Here's the drawing with two shaded views (mm, measured from the low corner). I have some questions. A direction names the side the tool comes from. Coordinates: 2 decimals unless noted, no trailing zeros. Write each loop counter-clockwise with the first axis right and the second up, starting at its lowest first coordinate (ties: lowest second). Pieces come first, ordered by that corner, then holes. Notation, with made-up numbers: (23, 38.5) -> (79, 38.5) arc R27 ccw to (79, 65.5) -> close; hole circle Ø6 at (11.5, -33). An arc over 180 degrees is marked (long way). Answer in a Markdown table with one row per item. Add a question column.
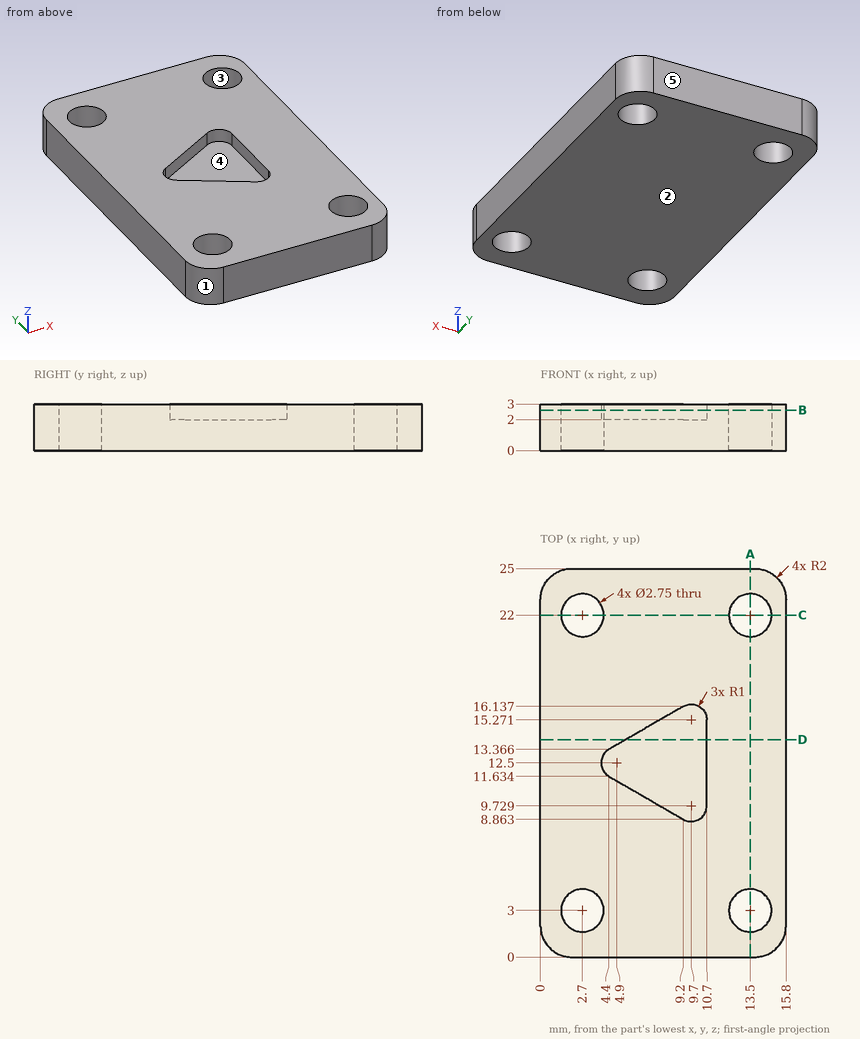
Q1. Imagine slicing it at C-C on y = 22. Please give me the cut outline in (x, z) (1 decimal).
Q2. Imagine slicing it at A-A on x = 13.5. Please give me the cut outline in (y, z) (1 decimal), plus the area to 3 significant figures.
Q3. For the marked faces 4 and 5, which set-ups out of +Z, -Z, +X, -X, +Y, -Y let a thin tool reach every point of the face, with its end or its side?
Q4. I'm going to push a flat-ended pin straight in: P1, Ø1.6, axis at x = 13.5, y = 3, coming from the -Z side. Where does the tip first touch, or does it pass through?
Q5. Imagine slicing it at B-B on z = 2.6. State how many separate pieces and enclosed holes the cut face has, plus the area to 3 significant figures.
Q6. I need wall thicknesses on line 1 (Y direction, x = 2.7, z = 1.8) (1 decimal); line 2 (Y direction, x = 2.25, z = 1.5); line 3 (X direction, y = 23.25, z = 0.4) (1 decimal). Which ranges of each line are inside material? Lowest first, please. Write a range as [from, to].
Q7. Imagine slicing it at D-D on y = 14. Please give me the cut outline in (x, z).
Q8. If we mould it in two halves opening along Y, with no side actions, what happens to the marked faces 1, 2 and 3? For each: pulls with the +Y half, pulls with the -Y half, needs draft (parallel to the pull), parting line crosses it, or undercut.
Result sheet:
| question | item | result |
|---|---|---|
| 1 | outline | (0, 0) -> (1.3, 0) -> (1.3, 3) -> (0, 3) -> close; (4.1, 0) -> (12.1, 0) -> (12.1, 3) -> (4.1, 3) -> close; (14.9, 0) -> (15.8, 0) -> (15.8, 3) -> (14.9, 3) -> close |
| 2 | outline | (0, 0) -> (1.6, 0) -> (1.6, 3) -> (0, 3) -> close; (4.4, 0) -> (20.6, 0) -> (20.6, 3) -> (4.4, 3) -> close; (23.4, 0) -> (25, 0) -> (25, 3) -> (23.4, 3) -> close |
| 2 | area | 58.5 mm^2 |
| 3 | face 4 | +Z |
| 3 | face 5 | +Z, -Z, +X, -X, +Y |
| 4 | P1 | passes through |
| 5 | separate pieces | 1 |
| 5 | enclosed holes | 5 |
| 5 | area | 335 mm^2 |
| 6 | line 1 | y = [0, 1.6], [4.4, 20.6], [23.4, 25] |
| 6 | line 2 | y = [0, 1.7], [4.3, 20.7], [23.3, 25] |
| 6 | line 3 | x = [0, 2.1], [3.3, 12.9], [14.1, 15.8] |
| 7 | outline | (0, 0) -> (15.8, 0) -> (15.8, 3) -> (10.7, 3) -> (10.7, 2) -> (5.5, 2) -> (5.5, 3) -> (0, 3) -> close |
| 8 | face 1 | pulls with the -Y half |
| 8 | face 2 | needs draft |
| 8 | face 3 | undercut |
